Autodesk Inventor part; units mm, degrees
ref_plane "YZ Plane" through (0, 0, 0) normal (1, 0, 0) x (0, 1, 0)
ref_plane "XZ Plane" through (0, 0, 0) normal (0, 1, 0) x (-1, 0, 0)
ref_plane "XY Plane" through (0, 0, 0) normal (0, 0, 1) x (1, 0, 0)
sketch "Sketch1" plane through (0, 0, 0) normal (1, 0, 0) x (0, 1, 0)
  line L0 (0, 0) -> (69.85, 0)
  line L1 (69.85, 0) -> (69.85, -150.4)
  line L2 (69.85, -150.4) -> (0, -150.4)
  line L3 (0, -150.4) -> (0, 0)
  dimension "d0" = 69.85
  dimension "d1" = 150.4
extrude "Extrusion1" add sketch "Sketch1" along normal blind 2
sketch "Sketch2" plane through (2, 0, 0) normal (1, 0, 0) x (0, 0, -1)
  line L0 (150.4, 0) -> (150.4, 69.85)
  line L1 (150.4, 69.85) -> (0, 69.85)
  line L2 (0, 69.85) -> (0, 0)
  line L3 (0, 0) -> (150.4, 0)
  line L4 (150.4, 69.85) -> (148.4, 69.85)
  line L5 (148.4, 69.85) -> (148.4, 0)
  line L6 (148.4, 0) -> (150.4, 0)
  line L7 (150.4, 0) -> (150.4, 69.85)
  line L8 (0, 69.85) -> (2, 69.85)
  line L9 (2, 69.85) -> (2, 0)
  line L10 (2, 0) -> (0, 0)
  line L11 (0, 0) -> (0, 69.85)
  line L12 (0, 0) -> (150.4, 0)
  line L13 (150.4, 0) -> (150.4, 2)
  line L14 (150.4, 2) -> (0, 2)
  line L15 (0, 2) -> (0, 0)
  point P0 (2, 2)
  point P1 (148.4, 2)
  dimension "d4" = 2
  dimension "d5" = 2
  dimension "d6" = 2
extrude "Extrusion2" add sketch "Sketch2" along normal blind 2 contours L14 L9 L1 L5
sketch "Sketch3" plane through (4, 0, 0) normal (1, 0, 0) x (0, 0, -1)
  line L0 (150.4, 0) -> (150.4, 69.85)
  line L1 (0, 0) -> (150.4, 0)
  line L2 (0, 69.85) -> (0, 0)
  line L3 (150.4, 69.85) -> (0, 69.85)
  line L4 (0, 69.85) -> (75.2, 69.85) construction
  line L5 (75.2, 69.85) -> (75.2, 0) construction
  line L6 (75.2, 0) -> (0, 0) construction
  line L7 (0, 0) -> (0, 69.85) construction
  line L8 (0, 0) -> (150.4, 0) construction
  line L9 (0, 0) -> (37.6, 0) construction
  line L10 (37.6, 0) -> (37.6, 69.85) construction
  line L11 (37.6, 69.85) -> (0, 69.85) construction
  line L12 (0, 69.85) -> (0, 0) construction
  line L13 (150.4, 0) -> (150.4, 69.85) construction
  line L14 (75.2, 69.85) -> (150.4, 69.85) construction
  line L15 (150.4, 69.85) -> (150.4, 0) construction
  line L16 (150.4, 0) -> (75.2, 0) construction
  line L17 (75.2, 0) -> (75.2, 69.85) construction
  line L18 (75.2, 0) -> (112.8, 0) construction
  line L19 (112.8, 0) -> (112.8, 69.85) construction
  line L20 (112.8, 69.85) -> (75.2, 69.85) construction
  line L21 (75.2, 69.85) -> (75.2, 0) construction
  line L22 (34.425, 0) -> (34.425, 69.85) construction
  line L23 (34.425, 69.85) -> (40.775, 69.85) construction
  line L24 (40.775, 69.85) -> (40.775, 0) construction
  line L25 (40.775, 0) -> (34.425, 0) construction
  line L26 (34.425, 0) -> (40.775, 69.85) construction
  line L27 (34.425, 69.85) -> (40.775, 0) construction
  line L28 (72.025, 0) -> (72.025, 69.85) construction
  line L29 (72.025, 69.85) -> (78.375, 69.85) construction
  line L30 (78.375, 69.85) -> (78.375, 0) construction
  line L31 (78.375, 0) -> (72.025, 0) construction
  line L32 (72.025, 0) -> (78.375, 69.85) construction
  line L33 (72.025, 69.85) -> (78.375, 0) construction
  line L34 (109.625, 0) -> (109.625, 69.85) construction
  line L35 (109.625, 69.85) -> (115.975, 69.85) construction
  line L36 (115.975, 69.85) -> (115.975, 0) construction
  line L37 (115.975, 0) -> (109.625, 0) construction
  line L38 (109.625, 0) -> (115.975, 69.85) construction
  line L39 (109.625, 69.85) -> (115.975, 0) construction
  line L40 (34.425, 69.85) -> (40.775, 69.85)
  line L41 (40.775, 69.85) -> (40.775, 0)
  line L42 (40.775, 0) -> (34.425, 0)
  line L43 (34.425, 0) -> (34.425, 69.85)
  line L44 (72.025, 0) -> (78.375, 0)
  line L45 (78.375, 0) -> (78.375, 69.85)
  line L46 (78.375, 69.85) -> (72.025, 69.85)
  line L47 (72.025, 69.85) -> (72.025, 0)
  line L48 (109.625, 69.85) -> (115.975, 69.85)
  line L49 (115.975, 69.85) -> (115.975, 0)
  line L50 (115.975, 0) -> (109.625, 0)
  line L51 (109.625, 0) -> (109.625, 69.85)
  point P0 (37.6, 34.925)
  point P1 (75.2, 34.925)
  point P2 (112.8, 34.925)
  dimension "d9" = 6.35
  dimension "d10" = 6.35
  dimension "d11" = 6.35
extrude "Extrusion3" add sketch "Sketch3" along normal blind 4 contours L1 L51 L3 L49 | L1 L47 L3 L45 | L1 L43 L3 L41
sketch "Sketch4" plane through (0, 69.85, 0) normal (0, 1, 0) x (1, 0, 0)
  line L0 (0, 150.4) -> (0, 0)
  line L1 (0, 150.4) -> (0, 0) construction
  line L2 (0, 0) -> (2, 0) construction
  line L3 (2, 2) -> (2, 0) construction
  line L4 (2, 2) -> (4, 2) construction
  line L5 (4, 34.425) -> (4, 2) construction
  line L6 (4, 34.425) -> (8, 34.425) construction
  line L7 (8, 40.775) -> (8, 34.425) construction
  line L8 (4, 40.775) -> (8, 40.775) construction
  line L9 (4, 72.025) -> (4, 40.775) construction
  line L10 (4, 72.025) -> (8, 72.025) construction
  line L11 (8, 78.375) -> (8, 72.025) construction
  line L12 (4, 78.375) -> (8, 78.375) construction
  line L13 (4, 109.625) -> (4, 78.375) construction
  line L14 (4, 109.625) -> (8, 109.625) construction
  line L15 (8, 115.975) -> (8, 109.625) construction
  line L16 (4, 115.975) -> (8, 115.975) construction
  line L17 (4, 148.4) -> (4, 115.975) construction
  line L18 (2, 148.4) -> (4, 148.4) construction
  line L19 (2, 150.4) -> (2, 148.4) construction
  line L20 (0, 150.4) -> (2, 150.4) construction
  line L21 (2, 0) -> (0, 0)
  line L22 (0, 0) -> (0, 150.4)
  line L23 (0, 150.4) -> (2, 150.4)
  line L24 (2, 150.4) -> (2, 0)
  line L25 (2, 0) -> (8, 0)
  line L26 (8, 0) -> (8, 150.4)
  line L27 (8, 150.4) -> (2, 150.4)
  line L28 (2, 150.4) -> (2, 0)
extrude "Extrusion4" cut sketch "Sketch4" against normal blind 2 contours L27 L26 L25 L24
sketch "Sketch5" plane through (0, 67.85, 0) normal (0, 1, 0) x (1, 0, 0)
  line L0 (4, 115.975) -> (8, 115.975)
  line L1 (4, 148.4) -> (4, 115.975)
  line L2 (2, 148.4) -> (4, 148.4)
  line L3 (2, 2) -> (2, 148.4)
  line L4 (4, 2) -> (2, 2)
  line L5 (4, 34.425) -> (4, 2)
  line L6 (8, 34.425) -> (4, 34.425)
  line L7 (8, 40.775) -> (8, 34.425)
  line L8 (4, 40.775) -> (8, 40.775)
  line L9 (4, 72.025) -> (4, 40.775)
  line L10 (8, 72.025) -> (4, 72.025)
  line L11 (8, 78.375) -> (8, 72.025)
  line L12 (4, 78.375) -> (8, 78.375)
  line L13 (4, 109.625) -> (4, 78.375)
  line L14 (8, 109.625) -> (4, 109.625)
  line L15 (8, 115.975) -> (8, 109.625)
  line L16 (2, 2) -> (4, 2)
  line L17 (2, 2) -> (8, 2)
  line L18 (8, 2) -> (8, 148.4)
  line L19 (8, 148.4) -> (2, 148.4)
  line L20 (2, 148.4) -> (2, 2)
  point P0 (0, 0)
  point P1 (4, 2)
extrude "Extrusion5" add sketch "Sketch5" against normal blind 2 contours L1 L19 L18 L0 | L18 L12 L13 L14 | L18 L8 L9 L10 | L5 L6 L18 L17
sketch "Sketch7" plane through (4, 0, 0) normal (-1, 0, 0) x (0, 0, 1)
  line L0 (-109.625, 2) -> (-115.975, 2)
  line L1 (-115.975, 0) -> (-115.975, 2)
  line L2 (-109.625, 0) -> (-115.975, 0)
  line L3 (-109.625, 2) -> (-109.625, 0)
  line L4 (-72.025, 2) -> (-78.375, 2)
  line L5 (-78.375, 0) -> (-78.375, 2)
  line L6 (-72.025, 0) -> (-78.375, 0)
  line L7 (-72.025, 2) -> (-72.025, 0)
  line L8 (-34.425, 2) -> (-40.775, 2)
  line L9 (-40.775, 0) -> (-40.775, 2)
  line L10 (-34.425, 0) -> (-40.775, 0)
  line L11 (-34.425, 2) -> (-34.425, 0)
  point P0 (0, 0)
extrude "Extrusion6" add sketch "Sketch7" along normal blind 2
sketch "Sketch8" plane through (0, 67.85, 0) normal (0, 1, 0) x (1, 0, 0)
  line L0 (8, 2) -> (8, 148.4) construction
  line L1 (2, 148.4) -> (8, 148.4) construction
  line L2 (2, 2) -> (2, 148.4) construction
  line L3 (8, 2) -> (2, 2) construction
  line L4 (8, 34.425) -> (2, 34.425) construction
  line L5 (2, 34.425) -> (2, 40.775) construction
  line L6 (2, 40.775) -> (8, 40.775) construction
  line L7 (8, 40.775) -> (8, 34.425) construction
  circle A0 centre (5, 37.6) radius 2.25 construction
  line L8 (2, 2) -> (2, 148.4) construction
  line L9 (8, 109.625) -> (2, 109.625) construction
  line L10 (2, 109.625) -> (2, 115.975) construction
  line L11 (2, 115.975) -> (8, 115.975) construction
  line L12 (8, 115.975) -> (8, 109.625) construction
  circle A1 centre (5, 112.8) radius 2.25 construction
  circle A2 centre (5, 37.6) radius 2.25
  circle A3 centre (5, 112.8) radius 2.25
  point P0 (0, 0)
  point P1 (8, 72.025)
  point P2 (8, 78.375)
  dimension "d20" = 4.5
  dimension "d21" = 4.5
extrude "Extrusion7" cut sketch "Sketch8" against normal blind 5
sketch "Sketch9" plane through (0, 69.85, 0) normal (0, 1, 0) x (1, 0, 0)
  line L0 (-2.5975, -3.6239) -> (10.7707, -3.6239)
  line L1 (10.7707, -3.6239) -> (10.7707, 152.0694)
  line L2 (10.7707, 152.0694) -> (-2.5975, 152.0694)
  line L3 (-2.5975, 152.0694) -> (-2.5975, -3.6239)
  point P0 (0, 0)
extrude "Extrusion8" cut sketch "Sketch9" against normal blind 61.9125
properties part number "leftwall"
Geometry: final body of the model. Coordinates: model frame, mm. A direction names the side the tool comes from. Round coordinates to 2 decimals unless told otherwise and drop trailing zeros. Loops run counter-clockwise (first coordinate to the right, second up) from the corner with the lowest first, then second, coordinate; pieces in that order, holes last. Notation, with made-up numbers: M -16,56.5 L 40,56.5 A25 ccw 40,69.5 Z; hole C 54,20.5 d6. An arc over 180 degrees is marked long. One line per question, with ' | ' between items.
(1) Contact query for flat-ended pins moving along their axis: P1, Ø1.8, axis at y = 5.5, z = -93, coming from the +X side; P2, Ø1.6, axis at x = 3.5, z = -89.5, coming from the -Y side; P3, Ø1, axis at x = 5, y = 4, coming from the -Z side (3 decimals). Output: stop coordinate, or through.
Check result:
P1: stops at x = 4 | P2: stops at y = 2 | P3: stops at z = -115.975
(2) Cut plane C-C on z = -13.5. Return the cut outline in (x, y), plus the area to 4 significant figures.
Check result:
outline: M 0,0 L 2,0 L 2,2 L 4,2 L 4,7.94 L 0,7.94 Z | area: 27.75 mm2
(3) Pull-direction query (Z, two-part tool) for faces 4 (the flat face through (4, 5, -56)), 5 (the flat face through (0, 4, -74)); classes: +Z half, -Z half, draft (parallel to the pull), parting line (faces both ways), or undercut.
Check result:
face 4: undercut | face 5: draft
(4) Material intervals for line 1 along Z through (x, y) = (6, 6) (3 decimals); line 2 along X through (y, z) = (1.5, -55); line 3 along X through (y, z) = (2.25, -8), sorted ascending. Write a range as from..to.
Check result:
line 1: z = -115.975..-109.625, -78.375..-72.025, -40.775..-34.425 | line 2: x = 0..2 | line 3: x = 0..4
(5) Cut plane B-B on y = 4. Return the cut outline in (x, z) (3 decimals), plus the area to 3 significant figures.
Check result:
outline: M 0,-150.4 L 2,-150.4 L 2,-148.4 L 4,-148.4 L 4,-115.975 L 8,-115.975 L 8,-109.625 L 4,-109.625 L 4,-78.375 L 8,-78.375 L 8,-72.025 L 4,-72.025 L 4,-40.775 L 8,-40.775 L 8,-34.425 L 4,-34.425 L 4,-2 L 2,-2 L 2,0 L 0,0 Z | area: 670 mm2
(6) Access query for faces 1 (the flat face through (4, 5, -132)), 2 (the flat face through (4, 5, -94)), 3 (the flat face through (4, 5, -18)). Directions: +Z, -Z, +X, -X, +Y, -Y. A direction counts if a zero-diameter tool reaches every point of the face in a straight line with its end or side. Return the directions, or none.
Check result:
face 1: -Z, +X, +Y, -Y | face 2: +X, +Y, -Y | face 3: +Z, +X, +Y, -Y
(7) Cut plane A-A on x = 5.5. Return the cut outline in (y, z) (1 decimal), plus the area to 3 significant figures.
Check result:
outline: M 0,-116 L 7.9,-116 L 7.9,-109.6 L 0,-109.6 Z; M 0,-78.4 L 7.9,-78.4 L 7.9,-72 L 0,-72 Z; M 0,-40.8 L 7.9,-40.8 L 7.9,-34.4 L 0,-34.4 Z | area: 151 mm2
